Can you work these out from the drawing? Everything is in mm from the part's minimum corner. A direction names the side the tool comes from. Coordinates: 2 decimals unless noted, no trailing zeros. Loops run counter-clockwise (first coordinate to the right, second up) from the corner with the lowest first, then second, coordinate; pieces in that order, holes last.
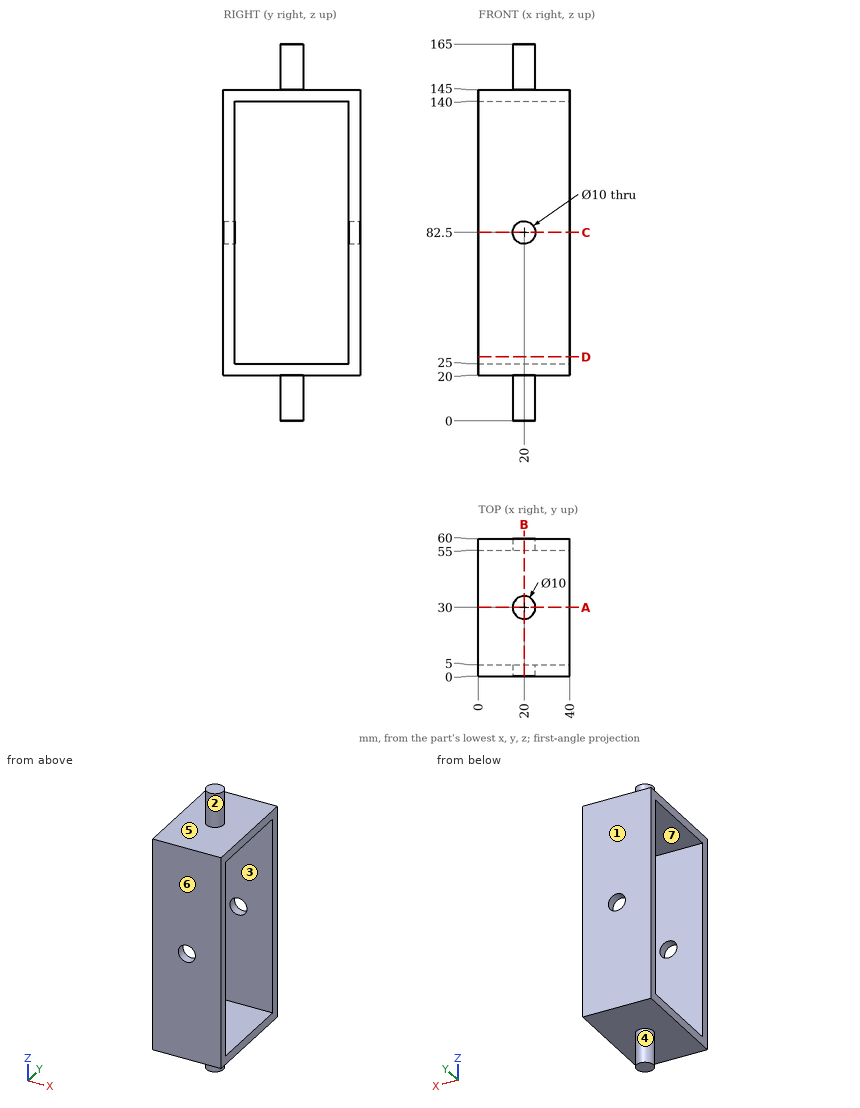
1) Imagine slicing it at A-A on y = 30. List the corners of the cut face in (x, z) for me, plus the area to 3 significant figures.
2) Will these pins go through, and if not, where does the flat tip stop? pin 1 (5 mm diameter, centred on x = 8, z = 86.5, fed in from -Y); pin 2 (2 mm diameter, centred on x = 4, y = 15, fed in from -Z); pin 3 (6 mm diameter, centred on x = 29.5, y = 30.5, fed in from +Z).
3) If I drill on L1, parallel to Y at x = 7, z = 48; L2, parallel to Z at x = 20, y = 1; L3, parallel to Z at x = 21.5, y = 54, over which ranges is the centre line in solid material (lowest first)?
4) Imagine slicing it at B-B on x = 20. List the corners of the cut face in (y, z) for me.
5) For the marked faces 1, 2, 3 and 4, which set-ups out of +Z, -Z, +X, -X, +Y, -Y let a thin tool reach every point of the face, with its end or its side?
6) Imagine slicing it at D-D on z = 28. List the corners of the cut face in (x, y) for me.
7) Imagine slicing it at C-C on z = 82.5. List the corners of the cut face in (x, y) for me.
8) We'd pull the mould along Z, two halves only. Please class the marked faces 5, 6 and 7: released by +Z, released by -Z, zero draft, split by the parting line, or undercut.
Solved:
1. outline: (0, 20) - (15, 20) - (15, 0) - (25, 0) - (25, 20) - (40, 20) - (40, 25) - (0, 25) - close; (0, 140) - (40, 140) - (40, 145) - (25, 145) - (25, 165) - (15, 165) - (15, 145) - (0, 145) - close
1. area: 800 mm2
2. pin 1: stops at y = 0
2. pin 2: stops at z = 20
2. pin 3: stops at z = 145
3. L1: y = 0 to 5, 55 to 60
3. L2: z = 20 to 77.5, 87.5 to 145
3. L3: z = 20 to 25, 140 to 145
4. outline: (0, 20) - (25, 20) - (25, 0) - (35, 0) - (35, 20) - (60, 20) - (60, 77.5) - (55, 77.5) - (55, 25) - (5, 25) - (5, 77.5) - (0, 77.5) - close; (0, 87.5) - (5, 87.5) - (5, 140) - (55, 140) - (55, 87.5) - (60, 87.5) - (60, 145) - (35, 145) - (35, 165) - (25, 165) - (25, 145) - (0, 145) - close
5. face 1: +Z, -Z, +X, -X, +Y
5. face 2: +Z
5. face 3: +X, -X
5. face 4: -Z
6. outline: (0, 0) - (40, 0) - (40, 5) - (0, 5) - close; (0, 55) - (40, 55) - (40, 60) - (0, 60) - close
7. outline: (0, 0) - (15, 0) - (15, 5) - (0, 5) - close; (0, 55) - (15, 55) - (15, 60) - (0, 60) - close; (25, 0) - (40, 0) - (40, 5) - (25, 5) - close; (25, 55) - (40, 55) - (40, 60) - (25, 60) - close
8. face 5: released by +Z
8. face 6: zero draft
8. face 7: undercut
